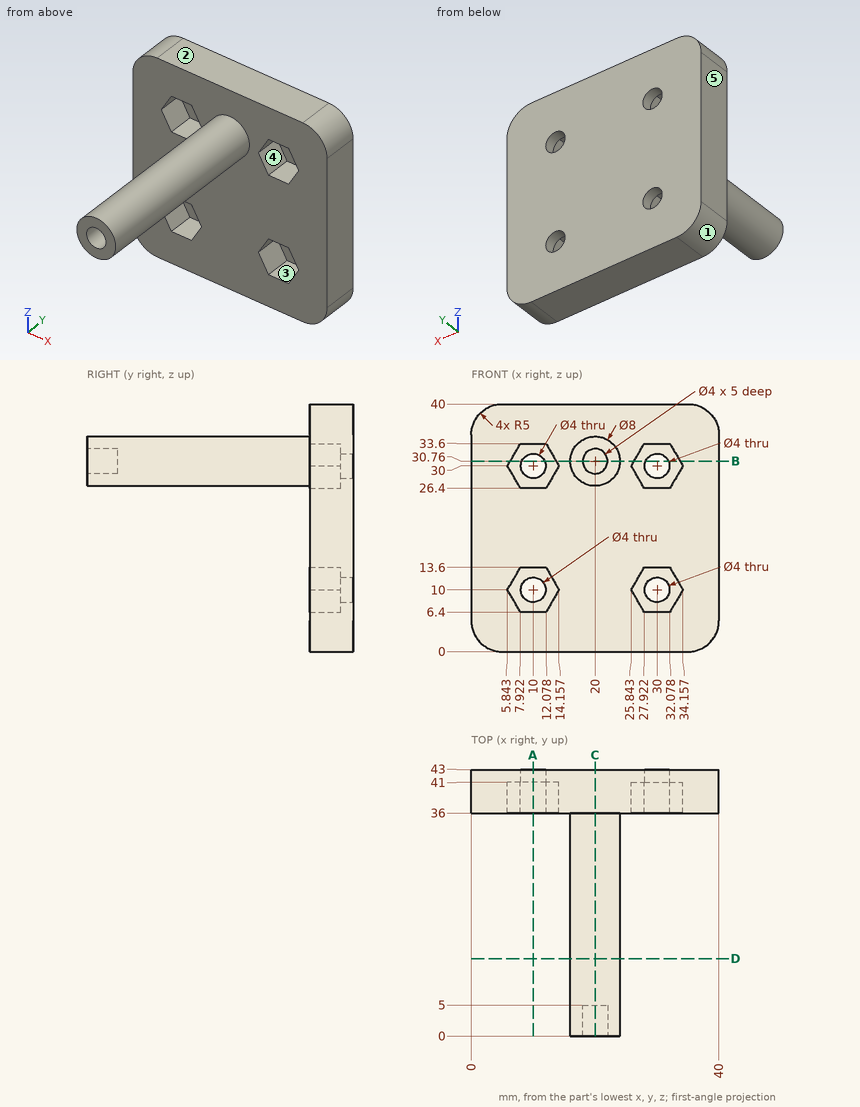
Here's the drawing with two shaded views (mm, measured from the low corner). I have some questions. A direction names the side the tool comes from. Coordinates: 2 decimals unless noted, no trailing zeros. Order: outer loops, then holes, each group sorted by start corner. A loop starts at its lowest first (then second) coordinate and runs counter-clockwise, first axis right, second up.
Item 1: If we section it at A-A, the plane x = 10: List the corners of the cut face in (y, z) for me, then the cut area to 3 significant figures.
Response values:
outline: (36, 0) - (43, 0) - (43, 8) - (41, 8) - (41, 6.4) - (36, 6.4) - close; (36, 13.6) - (41, 13.6) - (41, 12) - (43, 12) - (43, 28) - (41, 28) - (41, 26.4) - (36, 26.4) - close; (36, 33.6) - (41, 33.6) - (41, 32) - (43, 32) - (43, 40) - (36, 40) - close
area: 192 mm2
Item 2: If we section it at D-D, the plane y = 12.5: List the corners of the cut face in (x, z) for me.
Response values:
outline: circle Ø8 at (20, 30.76)
Item 3: I need wall thicknesses on probe 1 along Z at (x, y) = (10, 42); probe 2 along Z at (x, y) = (20, 1.2); probe 3 along Y at (x, z) = (33.5, 27). Which ranges of each line are inside material? Lowest first, please.
Response values:
probe 1: z = 0 to 8, 12 to 28, 32 to 40
probe 2: z = 26.76 to 28.76, 32.76 to 34.76
probe 3: y = 36 to 43
Item 4: Which directions (+Z, -Z, +X, -X, +Y, -Y) give clear straight access to the entire face, cutting with the end or side of a thin tool? Please do the marked faces 4 and 5.
Response values:
face 4: -Y
face 5: +Z, -Z, -X, +Y, -Y
Item 5: If we section it at B-B, the plane z = 30.76: List the corners of the cut face in (x, y) for me, then the cut area to 3 significant figures.
Response values:
outline: (0, 36) - (6.28, 36) - (6.28, 41) - (8.15, 41) - (8.15, 43) - (0, 43) - close; (11.85, 41) - (13.72, 41) - (13.72, 36) - (16, 36) - (16, 0) - (18, 0) - (18, 5) - (22, 5) - (22, 0) - (24, 0) - (24, 36) - (26.28, 36) - (26.28, 41) - (28.15, 41) - (28.15, 43) - (11.85, 43) - close; (31.85, 41) - (33.72, 41) - (33.72, 36) - (40, 36) - (40, 43) - (31.85, 43) - close
area: 459 mm2
Item 6: I'm going to push flat-ended pins straight in: pin 1 Ø2 at (x, y) = (30, 39.5) entering from -Z; pin 2 Ø1.2 at (x, z) = (20.5, 31) entering from -Y; pin 3 Ø8 at (x, y) = (29, 5) entering from -Z; pin 4 Ø12 at (x, z) = (28, 23) entering from -Y. Where does each tip first touch, or does it pass through?
Response values:
pin 1: stops at z = 0
pin 2: stops at y = 5
pin 3: passes through
pin 4: stops at y = 36
Item 7: Thinking about a two-plate mould opening in X: for the marked faces 1, 2 and 3, which applies, pulls with the +X half, pulls with the -X half, needs draft (parallel to the pull), parting line crosses it, or undercut?
Response values:
face 1: pulls with the -X half
face 2: needs draft
face 3: undercut
Item 8: If we section it at C-C, the plane x = 20: List the corners of the cut face in (y, z) for me.
Response values:
outline: (0, 26.76) - (36, 26.76) - (36, 0) - (43, 0) - (43, 40) - (36, 40) - (36, 34.76) - (0, 34.76) - (0, 32.76) - (5, 32.76) - (5, 28.76) - (0, 28.76) - close
